```python
from build123d import *

# Parameters (mm, degrees)
SKETCH1_R                 = 9.525
BOSS_EXTRUDE1_DEPTH       = 6.35
FILLET1_R                 = 3.175
F_6_CLEARANCE_HOLE1_D     = 3.7973
F_6_CLEARANCE_HOLE1_DEPTH = 6.35


with BuildPart() as part:
    # Sketch1 → Boss-Extrude1 (new body)
    with BuildSketch(Plane(origin=(0, 0, 0), x_dir=(0, 0, -1), z_dir=(1, 0, 0))):
        with BuildLine():
            Line((-19.05, 266.7), (19.05, 266.7))
            ThreePointArc((19.05, 266.7), (84.689584794, 151.864978949), (65.432294388, 21.003243067))
            Line((65.432294388, 21.003243067), (72.860995986, 15.649155186))
            Line((72.860995986, 15.649155186), (41.67338239, -27.623103343))
            Line((41.67338239, -27.623103343), (10.764626298, -5.346236488))
            Line((10.764626298, -5.346236488), (41.952239895, 37.92602204))
            Line((41.952239895, 37.92602204), (43.433779152, 39.981631379))
            ThreePointArc((43.433779152, 39.981631379), (53.452056919, 161.864823129), (-19.05, 260.35))
            Line((-19.05, 260.35), (-19.05, 266.7))
        make_face()
        with Locations((38.1, 0)):
            Circle(SKETCH1_R, mode=Mode.SUBTRACT)
    extrude(amount=BOSS_EXTRUDE1_DEPTH)

    # Fillet1
    fillet1_edges = [part.edges().sort_by_distance(p)[0] for p in [
        (3.175, 21.003243067, -65.432294388),
        (3.175, 15.649155186, -72.860995986),
        (3.175, -27.623103343, -41.67338239),
        (3.175, -5.346236488, -10.764626298),
        (3.175, 39.981631379, -43.433779152),
    ]]
    fillet(fillet1_edges, radius=FILLET1_R)

    # #6 Clearance Hole1
    with Locations(Plane(origin=(6.35, 0, 0), x_dir=(0, 0, -1), z_dir=(1, 0, 0))):
        with Locations((-15.875, 263.525), (15.875, 263.525), (0, 263.525)):
            Hole(F_6_CLEARANCE_HOLE1_D / 2, depth=F_6_CLEARANCE_HOLE1_DEPTH)


solid = part.part
```
The listing builds one solid part. Answer for the finished solid, in the listing's coordinates (mm). Coordinates: 2 decimals unless noted, no trailing zeros. Order: outer loops, then holes, each group sorted by start corner. A loop starts at its lowest first (then second) coordinate and runs counter-clockwise, first axis right, second up. Notation, with made-up numbers: M -6,15.25 L 49,15.25 A30 cw 49,37.25 Z; hole C 72.25,56 d3. An arc over 180 degrees is marked long. Answer as a JSON object with one key per item and string values. Group by question number.
1. Section B-B on x = 1.25 is taken. State how many separate pieces and enclosed holes the cut face has, then the cut area to 3 significant figures.
2. Straight lines are drawn through the part: line 1 (Y direction, x = 3.5, z = -38.1) (3 decimals); line 2 (Y direction, x = 6, z = -44.5); line 3 (Y direction, x = 5.5, z = -13). For each, find the intervals that lie inside material, in ascending order.
3. Section A-A on y = 0 is taken. Write down the section's boundary in (x, z) (3 decimals).
4. Section C-C on y = 84.5 is taken. Write down the section's boundary in (x, z), then the cut area to 3 significant figures.
5. Determine the mould class of faces 1 (the flat face through (6.35, 121, -63)), 2 (the flat face through (3.131, -16.615, -26.399)), 3 (the cylindrical face through (3.131, 0.419, -28.584)) for opening direction Z: released by +Z, released by -Z, zero draft, split by the parting line, or undercut.
6. Flat-ended cylindrical pins translate along their axes: P1, Ø1.5, axis at x = 5, y = 179.5, coming from the -Z side; P2, Ø2.5, axis at y = 263.525, z = 15.875, coming from the -X side. Find the tip coordinate at first contact, or state that the pin passes through.
7. Section D-D on z = -76 is taken. Write down the section's boundary in (x, y).
Values follow:
{
 "1": {"separate pieces": "1", "enclosed holes": "4", "area": "9,170 mm2"},
 "2": {"line 1": "-25.048 to -9.525, 9.525 to 32.581, 199.02 to 247.65", "line 2": "-23.7 to -7.05, 7.05 to 42.29, 186.31 to 239.96", "line 3": "-6.92 to -2.24, 233.45 to 266.7"},
 "3": {"outline": "M 0,-61.582 L 6.35,-61.582 L 6.35,-47.625 L 0,-47.625 Z; M 0,-28.575 L 6.35,-28.575 L 6.35,-14.618 L 0,-14.618 Z"},
 "4": {"outline": "M 0,-86 L 6.35,-86 L 6.35,-57.5 L 0,-57.5 Z", "area": "181 mm2"},
 "5": {"face 1": "zero draft", "face 2": "released by +Z", "face 3": "undercut"},
 "6": {"P1": "z = -77.67", "P2": "through"},
 "7": {"outline": "M 0,45.06 L 6.35,45.06 L 6.35,183.54 L 0,183.54 Z"}
}
